from build123d import *

# Parameters (mm, degrees)
F0_R     = 9.525
F0_R_2   = 12.7
F0_R_3   = 6.35
F1_DEPTH = 6.35
F2_R     = 12.7
F3_R     = 4.7625
F4_R     = 6.34999


# Not quite as in the source:
# - a fillet or chamfer is up to 0.001 mm smaller than in the source, because OpenCascade refuses the exact size


with BuildPart() as f1:
    # F0 (on Front) → F1 (new body, symmetric)
    with BuildSketch(Plane.XZ):
        with BuildLine():
            Line((-19.05, -60.325), (-19.05, -47.625))
            ThreePointArc((-19.05, -47.625), (0, -28.575), (19.05, -47.625))
            Line((19.05, -47.625), (19.05, -60.325))
            Line((19.05, -60.325), (44.45, -60.325))
            Line((44.45, -60.325), (44.45, -43.8458790377))
            ThreePointArc((44.45, -43.8458790377), (46.1544838519, -38.4084943559), (50.6579059691, -34.9171326425))
            Line((50.6579059691, -34.9171326425), (82.0025655956, -34.9171326425))
            ThreePointArc((82.0025655956, -34.9171326425), (101.6, -15.875), (82.0025655956, 3.1671326425))
            Line((82.0025655956, 3.1671326425), (82.55, 34.925))
            ThreePointArc((82.55, 34.925), (50.8, 66.675), (19.05, 34.925))
            Line((19.05, 34.925), (19.05, 28.575))
            Line((19.05, 28.575), (-19.05, 28.575))
            Line((-19.05, 28.575), (-19.05, 34.925))
            ThreePointArc((-19.05, 34.925), (-50.8, 66.675), (-82.55, 34.925))
            Line((-82.55, 34.925), (-82.0025655956, 3.1671326425))
            ThreePointArc((-82.0025655956, 3.1671326425), (-101.6, -15.875), (-82.0025655956, -34.9171326425))
            Line((-82.0025655956, -34.9171326425), (-50.6579059691, -34.9171326425))
            ThreePointArc((-50.6579059691, -34.9171326425), (-46.1544838519, -38.4084943559), (-44.45, -43.8458790377))
            Line((-44.45, -43.8458790377), (-44.45, -60.325))
            Line((-44.45, -60.325), (-19.05, -60.325))
        make_face()
        with Locations((-82.55, -15.875)):
            Circle(F0_R, mode=Mode.SUBTRACT)
        Circle(F0_R_2, mode=Mode.SUBTRACT)
        with Locations((82.55, -15.875)):
            Circle(F0_R, mode=Mode.SUBTRACT)
        with Locations((-50.8, 34.925)):
            Circle(F0_R_2, mode=Mode.SUBTRACT)
        with Locations((50.8, 34.925)):
            Circle(F0_R_2, mode=Mode.SUBTRACT)
        with Locations((82.55, -15.875)):
            Circle(F0_R)
        with Locations((82.55, -15.875)):
            Circle(F0_R_3, mode=Mode.SUBTRACT)
        with Locations((-82.55, -15.875)):
            Circle(F0_R)
        with Locations((-82.55, -15.875)):
            Circle(F0_R_3, mode=Mode.SUBTRACT)
    extrude(amount=F1_DEPTH, both=True)

    # F2
    f2_edges = [f1.edges().sort_by_distance(p)[0] for p in [
        (-44.45, 0, -60.325),
        (44.45, 0, -60.325),
    ]]
    fillet(f2_edges, radius=F2_R)

    # F3
    f3_edges = [f1.edges().sort_by_distance(p)[0] for p in [
        (-82.002566, 0, 3.167133),
        (82.002566, 0, 3.167133),
    ]]
    fillet(f3_edges, radius=F3_R)

    # F4 (radius 6.35 in the source; OpenCascade refuses exactly that, so slightly less here)
    f4_edges = [f1.edges().sort_by_distance(p)[0] for p in [
        (-19.05, 0, 28.575),
        (19.05, 0, 28.575),
    ]]
    fillet(f4_edges, radius=F4_R)


solid = f1.part
For this review, take the finished solid that the model builds, in its own axes (mm). A direction names the side the tool comes from. Round coordinates to 2 decimals unless told otherwise and drop trailing zeros. Loops run counter-clockwise (first coordinate to the right, second up) from the corner with the lowest first, then second, coordinate; pieces in that order, holes last. Notation, with made-up numbers: (-2, 32.25) - (6, 32.25) arc R10 cw to (6, 44.25) - close; hole circle Ø10 at (-18, -29). An arc over 180 degrees is marked (long way). One line per item, written item: value. Start each with the question number.
Item 1: For L1, parallel to Z at x = 50.8, y = 2.5 (3 decimals); L2, parallel to X at y = -4, z = 41; L3, parallel to X at y = 0, z = 29.5, list the stretches that pass through material, from the lowest coordinate up.
Item 2: The part is to be moulded in two halves that separate along Z. For faces 4 (the cylindrical face through (76.206, 0.089, -15.596)), 5 (the cylindrical face through (-83.19, 0.09, 4.49)), 6 (the flat face through (-44.45, 0, -46)), 7 (the flat face through (25, 0, -60.325)), say which applies: +Z half, -Z half, draft (parallel to the pull), parting line (faces both ways), or undercut.
Item 3: Take a section at C-C (y = 0.25). State how many separate pieces and enclosed holes the cut face has, plus the area to 3 significant figures.
Item 4: For faces 1 (the flat face through (19.05, 0, -54)), 2 (the cylindrical face through (83.19, -0.09, 4.49)), 3 (the cylindrical face through (17.14, 0.089, 30.386)), list the 3-axis set-ups (+Z, -Z, +X, -X, +Y, -Y) from which the entire face can be reached by the end or side of a thin tool; tool diameter is ignored.
Item 5: Take a section at D-D (z = 0). Give the boundary of the cut face in (x, y), plus the area to 3 significant figures.
Item 6: Take a section at A-A (x = 0). Give the boundary of the cut face in (y, z) (3 decimals).
Item 7: Clearance check with flat-ended pins moving along their axes: pin 1 Ø3 at (y, z) = (2, -46.5) entering from +X; pin 2 Ø4 at (y, z) = (-0.5, -56) entering from +X; pin 3 Ø1.5 at (y, z) = (3, -31.5) entering from +X. State where each tip first meets the part, or that it passes through.
Item 8: Take a section at B-B (z = 38). Give the boundary of the cut face in (x, y).
Answer below:
1. L1: z = -34.917 to 22.225, 47.625 to 66.675
1. L2: x = -81.96 to -61.95, -39.65 to -19.64, 19.64 to 39.65, 61.95 to 81.96
1. L3: x = -82.46 to -62.28, -39.32 to -16, 16 to 39.32, 62.28 to 82.46
2. face 4: undercut
2. face 5: undercut
2. face 6: draft
2. face 7: -Z half
3. separate pieces: 1
3. enclosed holes: 5
3. area: 15,000 mm2
4. face 1: -Z, +Y, -Y
4. face 2: +X, +Y, -Y
4. face 3: +Z, +Y, -Y
5. outline: (-93.08, -6.35) - (-12.7, -6.35) - (-12.7, 6.35) - (-93.08, 6.35) - close; (12.7, -6.35) - (93.08, -6.35) - (93.08, 6.35) - (12.7, 6.35) - close
5. area: 2,040 mm2
6. outline: (-6.35, -28.575) - (6.35, -28.575) - (6.35, -12.7) - (-6.35, -12.7) - close; (-6.35, 12.7) - (6.35, 12.7) - (6.35, 28.575) - (-6.35, 28.575) - close
7. pin 1: stops at x = 44.45
7. pin 2: stops at x = 42.73
7. pin 3: stops at x = 94.45
8. outline: (-82.4, -6.35) - (-63.12, -6.35) - (-63.12, 6.35) - (-82.4, 6.35) - close; (-38.48, -6.35) - (-19.2, -6.35) - (-19.2, 6.35) - (-38.48, 6.35) - close; (19.2, -6.35) - (38.48, -6.35) - (38.48, 6.35) - (19.2, 6.35) - close; (63.12, -6.35) - (82.4, -6.35) - (82.4, 6.35) - (63.12, 6.35) - close
